Input: part model. Units: mm. Frame: model coordinates. Face numbers are marked on the shaded views. Give positions to 0.01 mm unless a question says otherwise; leave off trailing zeros. Loops run counter-clockwise (first coordinate to the right, second up) from the corner with the lowest first, then second, coordinate; pieces in that order, holes last. Notation, with made-up numbers: (74, -32.5) -> (86, -32.5) arc R10 ccw to (86, -24.5) -> close; hole circle Ø11 at (61, -29). An arc over 180 degrees is marked (long way). One line per question, with ' | ' between items.
from build123d import *

# Parameters (mm, degrees)
CUT_EXTRUDE1_DEPTH = 0.75
FILLET1_R          = 0.125


with BuildPart() as part:
    # Sketch1 → Revolve1 (revolve)
    with BuildSketch(Plane(origin=(0, 0, 0), x_dir=(0, 0, -1), z_dir=(1, 0, 0))):
        with BuildLine():
            Line((0, 1.5), (-1.75, 1.5))
            ThreePointArc((-1.75, 1.5), (-2.334912942, 0.942930354), (-2.75, 0.25))
            Line((-2.75, 0.25), (-2.605662433, 0))
            Line((-2.605662433, 0), (-1.5, 0))
            Line((-1.5, 0), (-1.5, -20))
            Line((-1.5, -20), (0, -20))
            Line((0, -20), (0, 1.5))
        make_face()
    revolve(axis=Axis((0, -20, 0), (0, 1, 0)))

    # Sketch2 → Cut-Extrude1 (cut)
    with BuildSketch(Plane(origin=(0, 1.5, 0), x_dir=(1, 0, 0), z_dir=(0, 1, 0))):
        Polygon((0, 1.154700538), (-1, 0.577350269), (-1, -0.577350269), (0, -1.154700538), (1, -0.577350269), (1, 0.577350269), align=None)
    extrude(amount=-CUT_EXTRUDE1_DEPTH, mode=Mode.SUBTRACT)

    # Fillet1
    fillet1_edges = [part.edges().sort_by_distance(p)[0] for p in [
        (0.5, 1.5, -0.866025404),
        (-0.5, 1.5, -0.866025404),
        (-1, 1.5, 0),
        (-0.5, 1.5, 0.866025404),
        (0.5, 1.5, 0.866025404),
        (1, 1.5, 0),
        (0, 1.5, -1.75),
    ]]
    fillet(fillet1_edges, radius=FILLET1_R)


solid = part.part
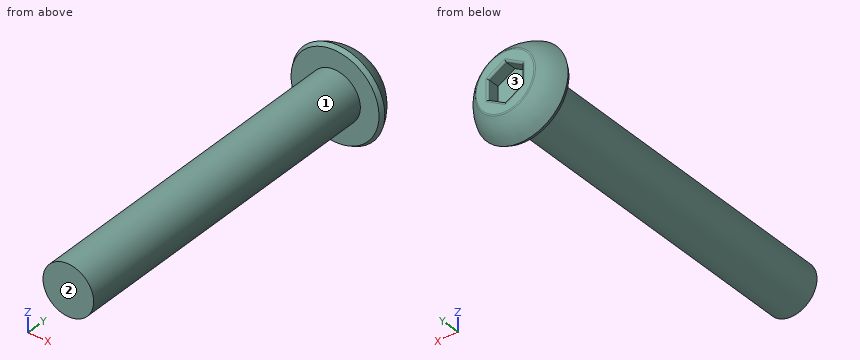
1. Pin query (flat end, axial travel): P1, Ø0.6, axis at x = 0, z = 0.5, coming from the +Y side; P2, Ø0.5, axis at y = 1, z = 0, coming from the +X side; P3, Ø1, axis at x = 0, y = -6.5, coming from the -Z side. Return the tip coordinate at first contact, or that it passes through.
Determined:
P1: stops at y = 0.75 | P2: stops at x = 2.48 | P3: stops at z = -1.5
2. Section query A-A (y = -16.75). Output: boundary loops of the cut face in (x, z), then the cut area to 3 significant figures.
Determined:
outline: circle Ø3 at (0, 0) | area: 7.07 mm2
3. Pull-direction query (X, two-part tool) for the marked faces 1, 2 and 3; classes: pulls with the +X half, pulls with the -X half, needs draft (parallel to the pull), parting line crosses it, or undercut.
Determined:
face 1: parting line crosses it | face 2: needs draft | face 3: undercut
4. Ray query, line 1 along X through (y, z) = (-7.5, 0.1); line 2 along Y through (x, z) = (-0.5, 0.15); line 3 along X through (y, z) = (-3.5, 1.35). Return the intervals inside material, ascending. Write a range as from..to.
Determined:
line 1: x = -1.5..1.5 | line 2: y = -20..0.75 | line 3: x = -0.65..0.65
